```python
from build123d import *

# Parameters (mm, degrees)
EXTRUDE_1_DEPTH     = 3
SKETCH_2_R          = 1.5
CUT_EXTRUDE_1_DEPTH = 10
SKETCH_3_W          = 10
SKETCH_3_H          = 172
SKETCH_3_W_2        = 90
SKETCH_3_H_2        = 33
EXTRUDE_2_DEPTH     = 3
SKETCH_4_R          = 1.6
CUT_EXTRUDE_2_DEPTH = 10
SKETCH_5_R          = 1.5
CUT_EXTRUDE_3_DEPTH = 10
SKETCH_6_R          = 1.5
CUT_EXTRUDE_4_DEPTH = 10
SKETCH_7_R          = 1.5
CUT_EXTRUDE_5_DEPTH = 74
SKETCH_8_R          = 1.5
CUT_EXTRUDE_6_DEPTH = 10
SKETCH_9_W          = 6
SKETCH_9_H          = 172
EXTRUDE_3_DEPTH     = 3
SKETCH_10_R         = 1.5
CUT_EXTRUDE_7_DEPTH = 15
CHAMFER_2_SIZE      = 2.5
CHAMFER_3_SIZE      = 2.5
CHAMFER_5_SIZE      = 2.5
SKETCH_11_R         = 1.5
CUT_EXTRUDE_8_DEPTH = 10
CHAMFER_6_SIZE      = 2
CHAMFER_7_SIZE      = 2
CHAMFER_8_SIZE      = 2


with BuildPart() as part:
    # 草图1 → 凸台-拉伸1 (new body)
    with BuildSketch(Plane.XY):
        Polygon((-105.75, 86), (-105.75, 70), (-105.75, -86), (105.75, -86), (105.75, 86), align=None)
    extrude(amount=EXTRUDE_1_DEPTH)

    # 草图2 → 切除-拉伸1 (cut)
    with BuildSketch(Plane.XY.offset(3)):
        with Locations((97.05, 83)):
            Circle(SKETCH_2_R)
        with Locations((-93.55, 83)):
            Circle(SKETCH_2_R)
        with Locations((57.55, 83)):
            Circle(SKETCH_2_R)
        with Locations((-54.05, 83)):
            Circle(SKETCH_2_R)
        with Locations((57.55, -83)):
            Circle(SKETCH_2_R)
        with Locations((97.05, -83)):
            Circle(SKETCH_2_R)
        with Locations((-54.05, -83)):
            Circle(SKETCH_2_R)
        with Locations((-93.55, -83)):
            Circle(SKETCH_2_R)
    extrude(amount=-CUT_EXTRUDE_1_DEPTH, mode=Mode.SUBTRACT)

    # 草图3 → 凸台-拉伸2 (add)
    with BuildSketch(Plane.XY.offset(3)):
        with Locations((110.75, 0)):
            Rectangle(SKETCH_3_W, SKETCH_3_H)
        with Locations((1.75, 99.5)):
            Rectangle(SKETCH_3_W_2, SKETCH_3_H_2)
        with Locations((1.75, -99.5)):
            Rectangle(SKETCH_3_W_2, SKETCH_3_H_2)
    extrude(amount=-EXTRUDE_2_DEPTH)

    # 草图4 → 切除-拉伸2 (cut)
    with BuildSketch(Plane.XY.offset(3)):
        with Locations((3.55, 34.3)):
            Circle(SKETCH_4_R)
        with Locations((47.31, 34.3)):
            Circle(SKETCH_4_R)
        with Locations((47.31, -34.3)):
            Circle(SKETCH_4_R)
        with Locations((3.55, -34.3)):
            Circle(SKETCH_4_R)
    extrude(amount=-CUT_EXTRUDE_2_DEPTH, mode=Mode.SUBTRACT)

    # 草图5 → 切除-拉伸3 (cut)
    with BuildSketch(Plane.XY.offset(3)):
        with Locations((92.75, 45)):
            Circle(SKETCH_5_R)
        with Locations((92.75, 25)):
            Circle(SKETCH_5_R)
        with Locations((92.75, -25)):
            Circle(SKETCH_5_R)
        with Locations((92.75, -45)):
            Circle(SKETCH_5_R)
    extrude(amount=-CUT_EXTRUDE_3_DEPTH, mode=Mode.SUBTRACT)

    # 草图6 → 切除-拉伸4 (cut)
    with BuildSketch(Plane.XY.offset(3)):
        with Locations((25.25, -89)):
            Circle(SKETCH_6_R)
        with Locations((-21.75, 89)):
            Circle(SKETCH_6_R)
        with Locations((25.25, 89)):
            Circle(SKETCH_6_R)
        with Locations((-21.75, -89)):
            Circle(SKETCH_6_R)
    extrude(amount=-CUT_EXTRUDE_4_DEPTH, mode=Mode.SUBTRACT)

    # 草图7 → 切除-拉伸5 (cut)
    with BuildSketch(Plane(origin=(0, 0, 0), x_dir=(-1, 0, 0), z_dir=(0, 0, -1))):
        with Locations((91.75, -60)):
            Circle(SKETCH_7_R)
        with Locations((91.75, -40)):
            Circle(SKETCH_7_R)
        with Locations((91.75, 60)):
            Circle(SKETCH_7_R)
        with Locations((91.75, 40)):
            Circle(SKETCH_7_R)
    extrude(amount=-CUT_EXTRUDE_5_DEPTH, mode=Mode.SUBTRACT)

    # 草图8 → 切除-拉伸6 (cut)
    with BuildSketch(Plane(origin=(0, 0, 0), x_dir=(-1, 0, 0), z_dir=(0, 0, -1))):
        with Locations((-97.75, 10)):
            Circle(SKETCH_8_R)
        with Locations((-97.75, -10)):
            Circle(SKETCH_8_R)
    extrude(amount=-CUT_EXTRUDE_6_DEPTH, mode=Mode.SUBTRACT)

    # 草图9 → 凸台-拉伸3 (add)
    with BuildSketch(Plane(origin=(0, 0, 0), x_dir=(-1, 0, 0), z_dir=(0, 0, -1))):
        with Locations((108.75, 0)):
            Rectangle(SKETCH_9_W, SKETCH_9_H)
    extrude(amount=-EXTRUDE_3_DEPTH)

    # 草图10 → 切除-拉伸7 (cut)
    with BuildSketch(Plane(origin=(0, 0, 0), x_dir=(-1, 0, 0), z_dir=(0, 0, -1))):
        with Locations((105.75, 76)):
            Circle(SKETCH_10_R)
        with Locations((105.75, 25)):
            Circle(SKETCH_10_R)
        with Locations((105.75, -25)):
            Circle(SKETCH_10_R)
        with Locations((105.75, -76)):
            Circle(SKETCH_10_R)
    extrude(amount=-CUT_EXTRUDE_7_DEPTH, mode=Mode.SUBTRACT)

    # 倒角2
    chamfer_2_edges = [part.edges().sort_by_distance(p)[0] for p in [
        (23.75, 89, 0),
    ]]
    chamfer(chamfer_2_edges, length=CHAMFER_2_SIZE)

    # 倒角3
    chamfer_3_edges = [part.edges().sort_by_distance(p)[0] for p in [
        (-23.25, 89, 0),
        (-90.25, -60, 0),
        (-90.25, -40, 0),
        (-90.25, 60, 0),
        (-90.25, 40, 0),
        (-104.25, 76, 0),
        (-104.25, 25, 0),
        (-104.25, -25, 0),
        (-104.25, -76, 0),
    ]]
    chamfer(chamfer_3_edges, length=CHAMFER_3_SIZE)

    # 倒角5
    chamfer_5_edges = [part.edges().sort_by_distance(p)[0] for p in [
        (91.25, 45, 0),
        (91.25, 25, 0),
        (91.25, -25, 0),
        (91.25, -45, 0),
        (99.25, 10, 0),
        (99.25, -10, 0),
    ]]
    chamfer(chamfer_5_edges, length=CHAMFER_5_SIZE)

    # 草图11 → 切除-拉伸8 (cut)
    with BuildSketch(Plane(origin=(0, 0, 0), x_dir=(-1, 0, 0), z_dir=(0, 0, -1))):
        with Locations((-89.209242617, 70.25)):
            Circle(SKETCH_11_R)
        with Locations((-99.209242617, 70.25)):
            Circle(SKETCH_11_R)
    cut_extrude_8 = extrude(amount=-CUT_EXTRUDE_8_DEPTH, mode=Mode.SUBTRACT)

    # 镜向2: 切除-拉伸8 across plane
    add(cut_extrude_8.mirror(Plane.ZX), mode=Mode.SUBTRACT)

    # 倒角6
    chamfer_6_edges = [part.edges().sort_by_distance(p)[0] for p in [
        (45.71, 34.3, 0),
    ]]
    chamfer(chamfer_6_edges, length=CHAMFER_6_SIZE)

    # 倒角7
    chamfer_7_edges = [part.edges().sort_by_distance(p)[0] for p in [
        (1.95, 34.3, 0),
        (45.71, -34.3, 0),
        (1.95, -34.3, 0),
        (90.709242617, 70.25, 0),
        (100.709242617, 70.25, 0),
        (90.709242617, -70.25, 0),
        (100.709242617, -70.25, 0),
    ]]
    chamfer(chamfer_7_edges, length=CHAMFER_7_SIZE)

    # 倒角8
    chamfer_8_edges = [part.edges().sort_by_distance(p)[0] for p in [
        (23.75, -89, 0),
        (-23.25, -89, 0),
    ]]
    chamfer(chamfer_8_edges, length=CHAMFER_8_SIZE)

    # 镜向1: 切除-拉伸8 across plane
    add(cut_extrude_8.mirror(Plane.ZX), mode=Mode.SUBTRACT)


solid = part.part
```
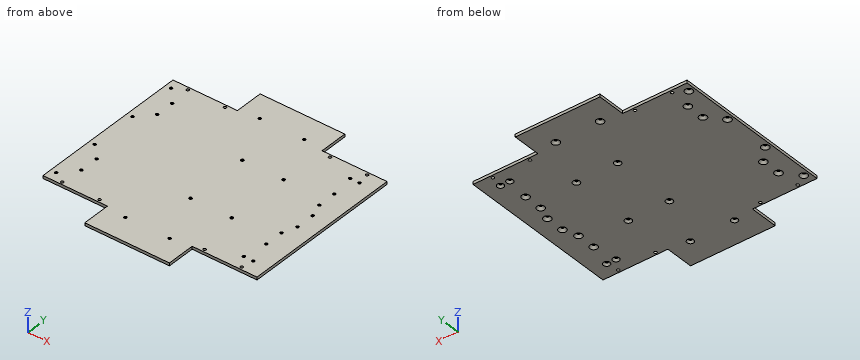
Input: part model. Units: mm. Frame: model coordinates. Give positions to 0.01 mm unless a question says otherwise; leave off trailing zeros. Order: outer loops, then holes, each group sorted by start corner. A loop starts at its lowest first (then second) coordinate and runs counter-clockwise, first axis right, second up. Notation, with made-up numbers: (-8, 9.5) - (16, 9.5) arc R24 ccw to (16, 27.5) - close; hole circle Ø5 at (-21, 85.5). An arc over 180 degrees is marked (long way). Use a Markdown table: item, result.
(1) Section query B-B (x = -74). Output: boundary loops of the cut face in (y, z), then the cut area to 3 significant figures.
Computed values:
| item | result |
|---|---|
| outline | (-86, 0) - (86, 0) - (86, 3) - (-86, 3) - close |
| area | 516 mm2 |
(2) Section query A-A (z = 0.55). State how many separate pieces and enclosed holes the cut face has, then the cut area to 3 significant figures.
Computed values:
| item | result |
|---|---|
| separate pieces | 1 |
| enclosed holes | 34 |
| area | 43,600 mm2 |
(3) Line query: line 1 (Y direction, x = 92.75, z = 2.8); line 2 (Y direction, x = -105.75, z = 2.85); line 3 (X direction, y = -89, z = 2.55). Output: solid intervals per line, ascending. Write a range as from..to.
Computed values:
| item | result |
|---|---|
| line 1 | y = -86..-46.5, -43.5..-26.5, -23.5..23.5, 26.5..43.5, 46.5..86 |
| line 2 | y = -86..-77.5, -74.5..-26.5, -23.5..23.5, 26.5..74.5, 77.5..86 |
| line 3 | x = -43.25..-23.25, -20.25..23.75, 26.75..46.75 |
(4) Pin query (flat end, axial travel): pin 1 (2.5 mm diameter, centred on x = 97.05, y = 83, fed in from +Z); pin 2 (0.9 mm diameter, centred on x = 96, z = 1.5, fed in from +Y); pin 3 (1.5 mm diameter, centred on y = -98.5, z = 1, fed in from +X). Return the tip coordinate at first contact, or that it passes through.
Computed values:
| item | result |
|---|---|
| pin 1 | passes through |
| pin 2 | stops at y = 86 |
| pin 3 | stops at x = 46.75 |
